Input: part model. Units: mm. Frame: model coordinates. Coordinates: 2 decimals unless noted, no trailing zeros. Loops run counter-clockwise (first coordinate to the right, second up) from the corner with the lowest first, then second, coordinate; pieces in that order, holes last. Notation, with made-up numbers: (35.5, -5.75) - (45.5, -5.75) arc R14 ccw to (45.5, 18.25) - close; hole circle Ø11 at (43.25, 2.25). An arc over 180 degrees is marked (long way). Use a Markdown table: item, result. Add a question column.
1. Ray query, L1, parallel to Z at x = -2.75, y = 3 (1 decimal); L2, parallel to Y at x = 0.5, z = 65; L3, parallel to Y at x = 3, z = 23.5. Return the intervals inside material, ascending. Write a range as [from, to].
2. Contact query for flat-ended pins moving along their axis: P1, Ø4, axis at y = -3.5, z = 53, coming from the -X side; P2, Ø5, axis at x = -2.5, z = 23, coming from the -Y side; P3, Ø0.7, axis at y = 4.5, z = 69.5, coming from the +X side; P4, Ø3, axis at y = 3.5, z = 90, coming from the -X side. Output: stop coordinate, or through.
3. Section query A-A on y = 2. Return the cut outline in (x, z) (1 decimal).
4. Section query B-B on z = 133. Return the cut outline in (x, y), then the cut area to 3 significant figures.
Autodesk Inventor part; units mm, degrees
ref_plane "Work Plane1" through (0, 0, 1.5875) normal (0, 0, -1) x (-1, 0, 0)
ref_plane "Work Plane2" through (0, 0, 130.683) normal (0, 0, -1) x (-1, 0, 0)
ref_plane "Work Plane3" through (0, 0, 153.9875) normal (0, 0, 1) x (1, 0, 0)
sketch "Sketch1" plane through (0, 0, 0) normal (0, 0, 1) x (1, 0, 0)
  arc A0 (-1, 4.6563) -> (1, 4.6563) centre (0, 0) ccw
  line L0 (-1, 3.7625) -> (1, 3.7625)
  line L1 (1, 3.7625) -> (1, 4.6563)
  line L2 (1, 5.7625) -> (-1, 5.7625) construction
  line L3 (-1, 5.7625) -> (-1, 4.6563) construction
  arc A1 (1, 4.6563) -> (-1, 4.6563) centre (0, 0) ccw construction
  line L4 (-1, 4.6563) -> (-1, 3.7625)
  line L5 (1, 4.6563) -> (1, 5.7625) construction
  dimension "d0" = 9.525
  dimension "d3" = 2
  dimension "d4" = 2
  dimension "d5" = 1
  dimension "d6" = 3.7625
extrude "Extrusion1" add sketch "Sketch1" along normal blind 155.575
ref_plane "Work Plane1" through (0, 0, 1.5875) normal (0, 0, -1) x (-1, 0, 0)
sketch "Sketch2" plane through (0, 0, 1.5875) normal (0, 0, -1) x (-1, 0, 0)
  line L0 (-1, 3.7625) -> (-1, 4.6563)
  line L1 (1, 3.7625) -> (-1, 3.7625)
  line L2 (1, 4.6563) -> (1, 3.7625)
  arc A0 (-1, 4.6563) -> (1, 4.6563) centre (0, 0) ccw
  arc A1 (-1, 3.8735) -> (1, 3.8735) centre (0, 0) ccw
  arc A2 (1, 3.8735) -> (-1, 3.8735) centre (0, 0) ccw construction
  dimension "d9" = 0.762
extrude "Extrusion2" cut sketch "Sketch2" against normal blind 0.762 contours A1 L2 A0 L0
ref_plane "Work Plane2" through (0, 0, 130.683) normal (0, 0, -1) x (-1, 0, 0)
sketch "Sketch3" plane through (0, 0, 130.683) normal (0, 0, -1) x (-1, 0, 0)
  arc A0 (-1, 3.8735) -> (1, 3.8735) centre (0, 0) ccw
  line L0 (-1, 3.7625) -> (-1, 4.6563)
  arc A1 (-1, 4.6563) -> (1, 4.6563) centre (0, 0) ccw
  line L1 (1, 4.6563) -> (1, 3.7625)
  line L2 (1, 3.7625) -> (-1, 3.7625)
extrude "Extrusion3" cut sketch "Sketch3" against normal blind 0.762 contours A0 L1 A1 L0
ref_plane "Work Plane3" through (0, 0, 153.9875) normal (0, 0, 1) x (1, 0, 0)
sketch "Sketch4" plane through (0, 0, 153.9875) normal (0, 0, 1) x (1, 0, 0)
  arc A0 (-1, 3.8735) -> (1, 3.8735) centre (0, 0) ccw
  line L0 (-1, 3.7625) -> (1, 3.7625)
  line L1 (-1, 4.6563) -> (-1, 3.7625)
  line L2 (1, 3.7625) -> (1, 4.6563)
  arc A1 (-1, 4.6563) -> (1, 4.6563) centre (0, 0) ccw
extrude "Extrusion4" cut sketch "Sketch4" against normal blind 1.016 contours A0 L2 A1 L1
equation "\"d4\" = d3"
properties part number "vertical drive shaft 3"
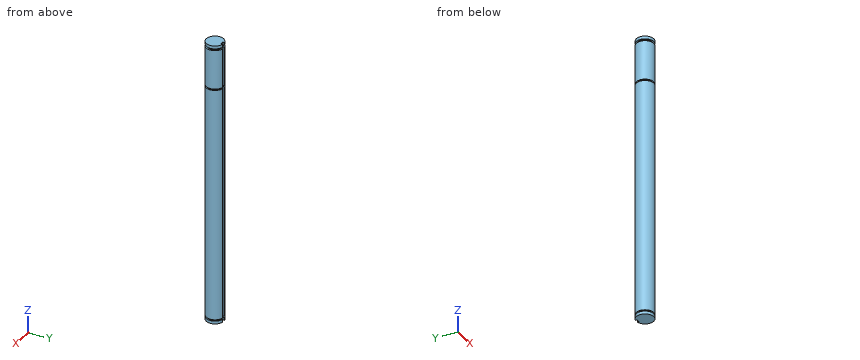
Resolved:
| question | item | result |
|---|---|---|
| 1 | L1 | [0, 1.6], [2.3, 130.7], [131.4, 153], [154, 155.6] |
| 1 | L2 | [-4.74, 3.76] |
| 1 | L3 | [-3.7, 3.7] |
| 2 | P1 | x = -4.52 |
| 2 | P2 | y = -4.76 |
| 2 | P3 | x = 2.34 |
| 2 | P4 | x = -4.32 |
| 3 | outline | (-4.3, 0) - (4.3, 0) - (4.3, 1.6) - (3.5, 1.6) - (3.5, 2.3) - (4.3, 2.3) - (4.3, 130.7) - (3.5, 130.7) - (3.5, 131.4) - (4.3, 131.4) - (4.3, 153) - (3.5, 153) - (3.5, 154) - (4.3, 154) - (4.3, 155.6) - (-4.3, 155.6) - (-4.3, 154) - (-3.5, 154) - (-3.5, 153) - (-4.3, 153) - (-4.3, 131.4) - (-3.5, 131.4) - (-3.5, 130.7) - (-4.3, 130.7) - (-4.3, 2.3) - (-3.5, 2.3) - (-3.5, 1.6) - (-4.3, 1.6) - close |
| 4 | outline | (-1, 3.76) - (-1, 4.66) arc R4.76 ccw (long way) to (1, 4.66) - (1, 3.76) - close |
| 4 | area | 69.3 mm² |
